from build123d import *

# Parameters (mm, degrees)
SKETCH_1_W      = 135
SKETCH_1_H      = 25
EXTRUDE_1_DEPTH = 5
SKETCH_3_W      = 105
SKETCH_3_H      = 5
EXTRUDE_2_DEPTH = 95
SKETCH_4_W      = 135
SKETCH_4_H      = 25
EXTRUDE_3_DEPTH = 5


with BuildPart() as part:
    # 草图1 → 凸台-拉伸1 (new body)
    with BuildSketch(Plane(origin=(0, 0, 0), x_dir=(0, 0, -1), z_dir=(1, 0, 0))):
        Rectangle(SKETCH_1_W, SKETCH_1_H)
    extrude(amount=EXTRUDE_1_DEPTH)

    # 草图3 → 凸台-拉伸2 (add)
    with BuildSketch(Plane(origin=(5, 0, 0), x_dir=(0, 0, -1), z_dir=(1, 0, 0))):
        with Locations((0, -10.300870967)):
            Rectangle(SKETCH_3_W, SKETCH_3_H)
    extrude(amount=EXTRUDE_2_DEPTH)

    # 草图4 → 凸台-拉伸3 (add)
    with BuildSketch(Plane(origin=(100, 0, 0), x_dir=(0, 0, -1), z_dir=(1, 0, 0))):
        Rectangle(SKETCH_4_W, SKETCH_4_H)
    extrude(amount=EXTRUDE_3_DEPTH)


solid = part.part
Build history of the part. All positions in model axes, mm. A direction names the side the tool comes from. Round coordinates to 2 decimals unless told otherwise and drop trailing zeros. Write each loop counter-clockwise with the first axis right and the second up, starting at its lowest first coordinate (ties: lowest second). Pieces come first, ordered by that corner, then holes. Notation, with made-up numbers: M -23,58.25 L 21,58.25 A31 ccw 21,90.25 Z; hole C -29,-22 d10. An arc over 180 degrees is marked long. Answer as a JSON object with one key per item and string values. Group by question number.
(1) Cut at A-A (y = 3). Give the cut face in (x, z), and give its area (3 significant figures).
(2) Drill centre lines: L1, parallel to X at y = 10.5, z = -15.5; L2, parallel to Y at x = 70, z = 34.5; L3, parallel to Z at x = 27, y = -9.5. Where is each one in solid material? Low to high.
(3) Mould opens along X. For faces 1 (the flat face through (0, 0, 1)), 2 (the flat face through (105, 0, 1)), 3 (the flat face through (2, 0, -67.5)), 4 (the flat face through (5, 3, 1)) say: pulls with the +X half, pulls with the -X half, needs draft (parallel to the pull), parting line crosses it, or undercut.
(4) Flat gauge pins, fed straight in: pin 1 (6 mm diameter, centred on x = 59.5, z = 0, fed in from +Y); pin 2 (4 mm diameter, centred on x = 50, y = -9.5, fed in from +Z); pin 3 (2.5 mm diameter, centred on x = 2.5, z = -14.5, fed in from -Y). Where does each tip first touch, or does it go through?
(5) Cut at D-D (x = 28.5). Give the cut face in (y, z), and give its area (3 significant figures).
(6) Cut at B-B (y = -10.25). Give the cut face in (x, z).
(7) Which spindle directions (+Z, -Z, +X, -X, +Y, -Y) get a long thin tool onto all of the face, cutting with end or side? Do faces 5 (the flat face through (2, -12.5, 1)), 6 (the flat face through (52, -7.801, 1)), 7 (the flat face through (102, -12.5, 1)). Say none if no direction does.
(8) Cut at C-C (z = -51). Give the cut face in (x, y), and give its area (3 significant figures).
Responses:
{
 "1": {"outline": "M 0,-67.5 L 5,-67.5 L 5,67.5 L 0,67.5 Z; M 100,-67.5 L 105,-67.5 L 105,67.5 L 100,67.5 Z", "area": "1,350 mm2"},
 "2": {"L1": "x = 0 to 5, 100 to 105", "L2": "y = -12.8 to -7.8", "L3": "z = -52.5 to 52.5"},
 "3": {"face 1": "pulls with the -X half", "face 2": "pulls with the +X half", "face 3": "needs draft", "face 4": "undercut"},
 "4": {"pin 1": "stops at y = -7.8", "pin 2": "stops at z = 52.5", "pin 3": "stops at y = -12.5"},
 "5": {"outline": "M -12.8,-52.5 L -7.8,-52.5 L -7.8,52.5 L -12.8,52.5 Z", "area": "525 mm2"},
 "6": {"outline": "M 0,-67.5 L 5,-67.5 L 5,-52.5 L 100,-52.5 L 100,-67.5 L 105,-67.5 L 105,67.5 L 100,67.5 L 100,52.5 L 5,52.5 L 5,67.5 L 0,67.5 Z"},
 "7": {"face 5": "+Z, -Z, -X, -Y", "face 6": "+Z, -Z, +Y", "face 7": "+Z, -Z, +X, -Y"},
 "8": {"outline": "M 0,-12.5 L 5,-12.5 L 5,-12.8 L 100,-12.8 L 100,-12.5 L 105,-12.5 L 105,12.5 L 100,12.5 L 100,-7.8 L 5,-7.8 L 5,12.5 L 0,12.5 Z", "area": "725 mm2"}
}
